from build123d import *

# Parameters (mm, degrees)
F0_R     = 29.967448
F1_DEPTH = 25.4
F2_R     = 5.08
F3_R     = 21.358851
F4_DEPTH = 12.7


with BuildPart() as f1:
    # F0 (on Front) → F1 (new body)
    with BuildSketch(Plane.XZ):
        Circle(F0_R)
    extrude(amount=F1_DEPTH)

    # F2
    f2_edges = [f1.edges().sort_by_distance(p)[0] for p in [
        (-29.967448, 0, 0),
        (-29.967448, -25.4, 0),
    ]]
    fillet(f2_edges, radius=F2_R)

    # F3 (on face) → F4 (cut, symmetric)
    with BuildSketch(Plane.XZ.offset(25.4)):
        Circle(F3_R)
    extrude(amount=F4_DEPTH, both=True, mode=Mode.SUBTRACT)


solid = f1.part
The model under review builds one solid part; all positions refer to its coordinate system, in mm. A direction names the side the tool comes from. Round coordinates to 2 decimals unless told otherwise and drop trailing zeros. Loops run counter-clockwise (first coordinate to the right, second up) from the corner with the lowest first, then second, coordinate; pieces in that order, holes last. Notation, with made-up numbers: (-40, 89.5) -> (19, 89.5) arc R14 cw to (19, 95.5) -> close; hole circle Ø7 at (53, -39). An arc over 180 degrees is marked (long way). One line per question, with ' | ' between items. Start each with the question number.
Item 1: For pin 1 (6 mm diameter, centred on x = -18.5, z = -22, fed in from -Y); pin 2 (2 mm diameter, centred on x = 20.5, y = -4, fed in from +Z); pin 3 (12 mm diameter, centred on x = 12, y = -15.5, fed in from +Z), all flat-tipped, find the tip position at first contact; note any pin that passes through.
Item 2: Add section B-B, the plane x = 0. Write out the cut boundary in (y, z).
Item 3: Add section C-C, the plane z = 0. Write out the cut boundary in (x, y), then the cut area to 3 significant figures.
Item 4: Draft analysis for pull direction X (two halves, no side actions). For faces 1 (the face through (-23.781, -12.593, -18.235)), 2 (the face through (0, -12.7, 0)), 3 (the face through (0, 0, 0)), state which applies: +X half, -X half, draft (parallel to the pull), parting line (faces both ways), or undercut.
Item 5: Machinability: for faces 4 (the face through (11.5, -19.1, 18)), 5 (the face through (11, -25.4, 19)), which of the approach directions +Z, -Z, +X, -X, +Y, -Y give a long, thin tool a straight path to every point of the face, cutting with its end or side? Answer none if there is none.
Item 6: Add section A-A, the plane y = -13.5. Write out the cut boundary in (x, z), then the cut area to 3 significant figures.
Item 7: Wall thickness on line 1 along Z through (x, y) = (0, -17.5); line 2 along Y through (x, z) = (5, 3); line 3 along X through (y, z) = (-19.5, 18): over which ranges is each line inside the solid? List them lowest first. Write a range as [from, to].
Item 8: Add section D-D, the plane y = -6.5. Write out the cut boundary in (x, z).
Return value:
1) pin 1: stops at y = -25.33 | pin 2: stops at z = 22.64 | pin 3: stops at z = 29.36
2) outline: (-25.4, -24.89) arc R5.08 ccw to (-20.32, -29.97) -> (-5.08, -29.97) arc R5.08 ccw to (0, -24.89) -> (0, 24.89) arc R5.08 ccw to (-5.08, 29.97) -> (-20.32, 29.97) arc R5.08 ccw to (-25.4, 24.89) -> (-25.4, 21.36) -> (-12.7, 21.36) -> (-12.7, -21.36) -> (-25.4, -21.36) -> close
3) outline: (-29.97, -20.32) arc R5.08 ccw to (-24.89, -25.4) -> (-21.36, -25.4) -> (-21.36, -12.7) -> (21.36, -12.7) -> (21.36, -25.4) -> (24.89, -25.4) arc R5.08 ccw to (29.97, -20.32) -> (29.97, -5.08) arc R5.08 ccw to (24.89, 0) -> (-24.89, 0) arc R5.08 ccw to (-29.97, -5.08) -> close | area: 958 mm2
4) face 1: parting line | face 2: undercut | face 3: draft
5) face 4: -Y | face 5: +Z, -Z, +X, -X, -Y
6) outline: circle Ø59.93 at (0, 0); hole circle Ø42.72 at (0, 0) | area: 1,390 mm2
7) line 1: z = [-29.97, -21.36], [21.36, 29.97] | line 2: y = [-12.7, 0] | line 3: x = [-23.96, -11.5], [11.5, 23.96]
8) outline: circle Ø59.93 at (0, 0)
